Verification items for the finished model (mm, model axes). A direction names the side the tool comes from. Round coordinates to 2 decimals unless told otherwise and drop trailing zeros. Order: outer loops, then holes, each group sorted by start corner. A loop starts at its lowest first (then second) coordinate and runs counter-clockwise, first axis right, second up. Notation, with made-up numbers: (5.5, 76) -> (46.5, 76) arc R22 ccw to (46.5, 113) -> close; hole circle Ø9 at (81, 14). An arc over 180 degrees is marked (long way). Write item = value, one per line. Start each with the question number.
from build123d import *

# Parameters (mm, degrees)
F0_W     = 81.4197
F0_H     = 51.0032
F1_DEPTH = 0.79375
F2_R     = 2.54
F3_W     = 76.0984
F3_H     = 45.72
F4_DEPTH = 1.778
F5_W     = 24.139271
F5_H     = 10.512263
F6_DEPTH = 1.778


with BuildPart() as f1:
    # F0 (on Top) → F1 (new body, symmetric)
    with BuildSketch(Plane.XY):
        Rectangle(F0_W, F0_H)
    extrude(amount=F1_DEPTH, both=True)

    # F2
    f2_edges = [f1.edges().sort_by_distance(p)[0] for p in [
        (40.70985, -25.5016, 0),
        (40.70985, 25.5016, 0),
        (-40.70985, -25.5016, 0),
        (-40.70985, 25.5016, 0),
    ]]
    fillet(f2_edges, radius=F2_R)

    # F3 (on face) → F4 (join)
    with BuildSketch(Plane(origin=(0, 0, -0.79375), x_dir=(1, 0, 0), z_dir=(0, 0, -1))):
        Rectangle(F3_W, F3_H)
    extrude(amount=F4_DEPTH)

    # F5 (on face) → F6 (join, through all)
    with BuildSketch(Plane(origin=(0, 0, -0.79375), x_dir=(1, 0, 0), z_dir=(0, 0, -1))):
        with Locations((16.741752, 21.900548)):
            Rectangle(F5_W, F5_H)
    extrude(amount=F6_DEPTH)


solid = f1.part
(1) Cross-section at B-B (y = 17). Enter the section's corners in (x, z), and give its area (3 significant figures).
(2) Draft check along Z on faces 4 (the flat face through (-1, -2, -2.572)), 5 (the flat face through (-1, 0, 0.794)), 6 (the flat face through (17, -27.157, -2)). Enter one of: +Z half, -Z half, draft (parallel to the pull), parting line (faces both ways), or undercut.
(3) Cross-section at A-A (x = -4). Enter the section's corners in (y, z).
(4) Depth check by flat-ended pin: pin 1 (0.8 mm diameter, centred on x = 12, y = -26.5, fed in from +Z); pin 2 (0.9 mm diameter, centred on y = -24.5, z = -1.5, fed in from +X); pin 3 (1.4 mm diameter, centred on x = 31.5, z = -2, fed in from -Y). Enter the tip coordinate at first touch or a pass-through.
(5) Scan lines: line 1 along Z through (x, y) = (-15, 23.5); line 2 along X through (y, z) = (-9.5, -0.95); line 3 along Y through (x, z) = (-27.5, -1.1). Record each from-to range of solid material in increasing order. Write a range as from..to.
(6) Set-up check for faces 1 (the flat face through (4.672, -25, -2)), 2 (the flat face through (17, -26, -0.794)), 3 (the flat face through (33, -22.86, -2)): record each of +Z, -Z, +X, -X, +Y, -Y from which the full face is reachable in a straight line by a thin tool's end or side.
Outcome:
q1.outline = (-40.71, -0.79) -> (-38.05, -0.79) -> (-38.05, -2.57) -> (38.05, -2.57) -> (38.05, -0.79) -> (40.71, -0.79) -> (40.71, 0.79) -> (-40.71, 0.79) -> close
q1.area = 265 mm^2
q2.face_4 = -Z half
q2.face_5 = +Z half
q2.face_6 = draft
q3.outline = (-25.5, -0.79) -> (-22.86, -0.79) -> (-22.86, -2.57) -> (22.86, -2.57) -> (22.86, -0.79) -> (25.5, -0.79) -> (25.5, 0.79) -> (-25.5, 0.79) -> close
q4.pin_1 = -0.79
q4.pin_2 = 28.81
q4.pin_3 = -22.86
q5.line_1 = -0.79..0.79
q5.line_2 = -38.05..38.05
q5.line_3 = -22.86..22.86
q6.face_1 = -Z, -X, -Y
q6.face_2 = +Z, +X, -X, -Y
q6.face_3 = -Z, +X, -Y
